from build123d import *

# Parameters (mm, degrees)
ESQUISSE1_R                  = 5.75
ESQUISSE1_R_2                = 1.6
BOSS_EXTRU_1_DEPTH           = 5
ESQUISSE2_R                  = 3
ENL_V_MAT_EXTRU_1_DEPTH      = 3
ESQUISSE3_R                  = 5.75
ESQUISSE3_R_2                = 4.5
ENL_V_MAT_EXTRU_2_DEPTH      = 3
BOSS_EXTRU_2_DEPTH           = 2
R_P_TITION_CIRCULAIRE1_COUNT = 2
ESQUISSE5_R                  = 0.75
ENL_V_MAT_EXTRU_3_DEPTH      = 3
R_P_TITION_CIRCULAIRE2_COUNT = 2
BOSS_EXTRU_3_DEPTH           = 3
R_P_TITION_CIRCULAIRE3_COUNT = 28
ESQUISSE7_R                  = 3
ESQUISSE7_R_2                = 1.6
ENL_V_MAT_EXTRU_4_DEPTH      = 1
ESQUISSE8_R                  = 4.7
ESQUISSE8_R_2                = 3.4
ENL_V_MAT_EXTRU_5_DEPTH      = 1


with BuildPart() as part:
    # Esquisse1 → Boss.-Extru.1 (new body)
    with BuildSketch(Plane.XY):
        Circle(ESQUISSE1_R)
        Circle(ESQUISSE1_R_2, mode=Mode.SUBTRACT)
    extrude(amount=BOSS_EXTRU_1_DEPTH)

    # Esquisse2 → Enlèv. mat.-Extru.1 (cut)
    with BuildSketch(Plane.XY.offset(5)):
        Circle(ESQUISSE2_R)
    extrude(amount=-ENL_V_MAT_EXTRU_1_DEPTH, mode=Mode.SUBTRACT)

    # Esquisse3 → Enlèv. mat.-Extru.2 (cut)
    with BuildSketch(Plane.XY.offset(5)):
        Circle(ESQUISSE3_R)
        Circle(ESQUISSE3_R_2, mode=Mode.SUBTRACT)
    extrude(amount=-ENL_V_MAT_EXTRU_2_DEPTH, mode=Mode.SUBTRACT)

    # Esquisse4 → Boss.-Extru.2 (add)
    with BuildSketch(Plane(origin=(0, 0, 0), x_dir=(-1, 0, 0), z_dir=(0, 0, -1))):
        with BuildLine():
            Line((-4.3, 3.817394399), (-2.475852955, 16.846629695))
            ThreePointArc((-2.475852955, 16.846629695), (0, 19), (2.475852955, 16.846629695))
            Line((2.475852955, 16.846629695), (4.3, 3.817394399))
            ThreePointArc((4.3, 3.817394399), (0, 5.75), (-4.3, 3.817394399))
        make_face()
    boss_extru_2 = extrude(amount=-BOSS_EXTRU_2_DEPTH)

    # Répétition circulaire1: Boss.-Extru.2 ×2 about axis
    r_p_tition_circulaire1_axis = Axis((0, 0, 0), (0, 0, 1))
    for i in range(1, R_P_TITION_CIRCULAIRE1_COUNT):
        add(boss_extru_2.rotate(r_p_tition_circulaire1_axis, i * 360 / R_P_TITION_CIRCULAIRE1_COUNT))

    # Esquisse5 → Enlèv. mat.-Extru.3 (cut)
    with BuildSketch(Plane(origin=(0, 0, 0), x_dir=(-1, 0, 0), z_dir=(0, 0, -1))):
        with Locations((0, 7)):
            Circle(ESQUISSE5_R)
        with Locations((0, 10)):
            Circle(ESQUISSE5_R)
        with Locations((0, 13)):
            Circle(ESQUISSE5_R)
        with Locations((0, 16)):
            Circle(ESQUISSE5_R)
    enl_v_mat_extru_3 = extrude(amount=-ENL_V_MAT_EXTRU_3_DEPTH, mode=Mode.SUBTRACT)

    # Répétition circulaire2: Enlèv. mat.-Extru.3 ×2 about axis
    r_p_tition_circulaire2_axis = Axis((0, 0, 0), (0, 0, 1))
    for i in range(1, R_P_TITION_CIRCULAIRE2_COUNT):
        add(enl_v_mat_extru_3.rotate(r_p_tition_circulaire2_axis, i * 360 / R_P_TITION_CIRCULAIRE2_COUNT), mode=Mode.SUBTRACT)

    # Esquisse6 → Boss.-Extru.3 (add)
    with BuildSketch(Plane.XY.offset(5)):
        Polygon((-0.3, 3), (0, 2.7), (0.3, 3), align=None)
    boss_extru_3 = extrude(amount=-BOSS_EXTRU_3_DEPTH)

    # Répétition circulaire3: Boss.-Extru.3 ×28 about axis
    r_p_tition_circulaire3_axis = Axis((0, 0, 0), (0, 0, 1))
    for i in range(1, R_P_TITION_CIRCULAIRE3_COUNT):
        add(boss_extru_3.rotate(r_p_tition_circulaire3_axis, i * 360 / R_P_TITION_CIRCULAIRE3_COUNT))

    # Esquisse7 → Enlèv. mat.-Extru.4 (cut)
    with BuildSketch(Plane(origin=(0, 0, 0), x_dir=(-1, 0, 0), z_dir=(0, 0, -1))):
        Circle(ESQUISSE7_R)
        Circle(ESQUISSE7_R_2, mode=Mode.SUBTRACT)
    extrude(amount=-ENL_V_MAT_EXTRU_4_DEPTH, mode=Mode.SUBTRACT)

    # Esquisse8 → Enlèv. mat.-Extru.5 (cut)
    with BuildSketch(Plane(origin=(0, 0, 0), x_dir=(-1, 0, 0), z_dir=(0, 0, -1))):
        Circle(ESQUISSE8_R)
        Circle(ESQUISSE8_R_2, mode=Mode.SUBTRACT)
    extrude(amount=-ENL_V_MAT_EXTRU_5_DEPTH, mode=Mode.SUBTRACT)


solid = part.part
For this review, take the finished solid that the model builds, in its own axes (mm). A direction names the side the tool comes from. Round coordinates to 2 decimals unless told otherwise and drop trailing zeros. Write each loop counter-clockwise with the first axis right and the second up, starting at its lowest first coordinate (ties: lowest second). Pieces come first, ordered by that corner, then holes. Notation, with made-up numbers: M 87.5,-38 L 134.5,-38 A27 ccw 134.5,-13 Z; hole C 12.5,4 d11. An arc over 180 degrees is marked long. Write item = value, one per line. Start each with the question number.
(1) We need section B-B (y = -7). Give the boundary of the cut face in (x, z).
(2) Clearance check with flat-ended pins moving along their axes: pin 1 Ø2.5 at (x, y) = (0, -10) entering from -Z; pin 2 Ø2.5 at (x, y) = (0, 13) entering from +Z; pin 3 Ø2.5 at (x, y) = (0, 0) entering from +Z (1 decimal); pin 4 Ø1.8 at (x, y) = (-1.5, -1) entering from -Z. State where each tip first meets the part, or that it passes through.
(3) We need section A-A (z = 0.5). Give the number of separate pieces and of enclosed holes in the cut face, then the cut area to 3 significant figures.
(4) For faces 1 (the face through (1.02, -4.59, 0.49)), 2 (the face through (0.163, 6.268, 0.986)), 3 (the face through (1.3, -1.3, 2)), list the 3-axis set-ups (+Z, -Z, +X, -X, +Y, -Y) from which the entire face can be reached by the end or side of a thin tool; tool diameter is ignored.
(5) For line 1 along X through (y, z) = (1, 0.75); line 2 along Y through (x, z) = (-1, 0.5); line 3 along Z through (x, y) = (-1.75, 4), list the stretches that pass through material, from the lowest coordinate up.
(6) We need section C-C (y = -13). Give the boundary of the cut face in (x, z).
Results found:
q1.outline = M -3.85,0 L -0.75,0 L -0.75,2 L -3.85,2 Z; M 0.75,0 L 3.85,0 L 3.85,2 L 0.75,2 Z
q2.pin_1 = 0
q2.pin_2 = 2
q2.pin_3 = through
q2.pin_4 = 1
q3.separate_pieces = 2
q3.enclosed_holes = 10
q3.area = 198 mm²
q4.face_1 = -Z
q4.face_2 = +Z, -Z
q4.face_3 = +Z
q5.line_1 = -5.66 to -4.59, -3.25 to -2.83, 2.83 to 3.25, 4.59 to 5.66
q5.line_2 = -18.79 to -4.59, -3.25 to -2.83, 2.83 to 3.25, 4.59 to 18.79
q5.line_3 = 1 to 5
q6.outline = M -3.01,0 L -0.75,0 L -0.75,2 L -3.01,2 Z; M 0.75,0 L 3.01,0 L 3.01,2 L 0.75,2 Z
